from build123d import *

# Parameters (mm, degrees)
SKETCH_5_R          = 1.5
EXTRUDE_4_DEPTH     = 31
SKETCH_6_W          = 3
SKETCH_6_H          = 1.5
CUT_EXTRUDE_2_DEPTH = 3
CUT_EXTRUDE_3_DEPTH = 1.5
EXTRUDE_5_DEPTH     = 5


with BuildPart() as part:
    # 草图5 → 凸台-拉伸4 (new body)
    with BuildSketch(Plane.XY):
        Circle(SKETCH_5_R)
    extrude(amount=EXTRUDE_4_DEPTH)

    # 草图6 → 切除-拉伸2 (cut)
    with BuildSketch(Plane.XY.offset(31)):
        with Locations((0, 0.75)):
            Rectangle(SKETCH_6_W, SKETCH_6_H)
    extrude(amount=-CUT_EXTRUDE_2_DEPTH, mode=Mode.SUBTRACT)

    # 草图7 → 切除-拉伸3 (cut)
    with BuildSketch(Plane(origin=(0, 0, 0), x_dir=(1, 0, 0), z_dir=(0, 1, 0))):
        Polygon((-1.5, -28), (0, -30.598076211), (1.5, -28), (1.5, -31), (-1.5, -31), align=None)
    extrude(amount=-CUT_EXTRUDE_3_DEPTH, mode=Mode.SUBTRACT)

    # 草图8 → 凸台-拉伸5 (add)
    with BuildSketch(Plane(origin=(0, 0, 0), x_dir=(1, 0, 0), z_dir=(0, 1, 0))):
        Polygon((0, -30.598076211), (1.5, -28), (-1.5, -28), align=None)
    extrude(amount=EXTRUDE_5_DEPTH)


solid = part.part
For this review, take the finished solid that the model builds, in its own axes (mm). A direction names the side the tool comes from. Give positions to 0.01 mm unless a question says otherwise; leave off trailing zeros. Order: outer loops, then holes, each group sorted by start corner. A loop starts at its lowest first (then second) coordinate and runs counter-clockwise, first axis right, second up. Notation, with made-up numbers: (58.5, 42) - (105.5, 42) arc R29 ccw to (105.5, 78) - close; hole circle Ø8 at (39, 52). An arc over 180 degrees is marked (long way). Answer as a JSON object with one key per item and string values. Group by question number.
Item 1: Take a section at A-A on z = 9. Give the boundary of the cut face in (x, y).
Item 2: Take a section at B-B on x = 0.6. Give the boundary of the cut face in (y, z), and give its area (3 significant figures).
Item 3: Wall thickness on line 1 along Z through (x, y) = (1.1, 4.25); line 2 along Z through (x, y) = (0.15, 1.25); line 3 along Y through (x, z) = (0.15, 24.5): over which ranges is each line inside the solid? List them lowest first.
Item 4: Clearance check with a flat-ended pin moving along its axis: pin 1 Ø1.5 at (x, y) = (-0.5, 3) entering from -Z. State where the tip first meets the part, or that it passes through.
Item 5: Take a section at D-D on y = -0.5. Give the boundary of the cut face in (x, z), and give its area (3 significant figures).
Item 6: Take a section at C-C on y = 4. Give the boundary of the cut face in (x, z), and give its area (3 significant figures).
Item 7: Machinability: for faces 1 (the cylindrical face through (-0.325, -1.464, 15.085)), 2 (the flat face through (0, 0, 0)), which of the approach directions +Z, -Z, +X, -X, +Y, -Y give a long, thin tool a straight path to every point of the face, cutting with its end or side? Answer none if there is none.
Reported:
{
 "1": {"outline": "circle Ø3 at (0, 0)"},
 "2": {"outline": "(-1.37, 0) - (1.37, 0) - (1.37, 28) - (5, 28) - (5, 29.56) - (-1.37, 29.56) - close", "area": "86.9 mm^2"},
 "3": {"line 1": "28 to 28.69", "line 2": "0 to 30.34", "line 3": "-1.49 to 1.49"},
 "4": {"pin 1": "z = 28"},
 "5": {"outline": "(-1.41, 0) - (1.41, 0) - (1.41, 28.15) - (0, 30.6) - (-1.41, 28.15) - close", "area": "83.1 mm^2"},
 "6": {"outline": "(-1.5, 28) - (1.5, 28) - (0, 30.6) - close", "area": "3.90 mm^2"},
 "7": {"face 1": "-Z", "face 2": "-Z, +X, -X, +Y, -Y"}
}
